```python
from build123d import *

# Parameters (mm, degrees)
SKETCH1_R           = 1.5
SKETCH1_R_2         = 7.5
SKETCH1_W           = 3
SKETCH1_H           = 10
BOSS_EXTRUDE1_DEPTH = 3


with BuildPart() as part:
    # Sketch1 → Boss-Extrude1 (new body)
    with BuildSketch(Plane.XY):
        with BuildLine():
            Line((-41.926461559, 19.115471746), (-34.926461559, -16.884528254))
            ThreePointArc((-34.926461559, -16.884528254), (-33.544217508, -19.207626568), (-31, -20.121049617))
            Line((-31, -20.121049617), (31, -20.121049617))
            ThreePointArc((31, -20.121049617), (33.544217508, -19.207626568), (34.926461559, -16.884528254))
            Line((34.926461559, -16.884528254), (41.926461559, 19.115471746))
            ThreePointArc((41.926461559, 19.115471746), (41.086576951, 22.42316789), (38, 23.878950383))
            Line((38, 23.878950383), (37.313708499, 23.878950383))
            ThreePointArc((37.313708499, 23.878950383), (35.004307422, 23.144936706), (33.542472333, 21.212283716))
            ThreePointArc((33.542472333, 21.212283716), (30.618802154, 17.346977735), (26, 15.878950383))
            Line((26, 15.878950383), (-26, 15.878950383))
            ThreePointArc((-26, 15.878950383), (-30.618802154, 17.346977735), (-33.542472333, 21.212283716))
            ThreePointArc((-33.542472333, 21.212283716), (-35.004307422, 23.144936706), (-37.313708499, 23.878950383))
            Line((-37.313708499, 23.878950383), (-38, 23.878950383))
            ThreePointArc((-38, 23.878950383), (-41.086576951, 22.42316789), (-41.926461559, 19.115471746))
        make_face()
        with Locations((38, 19.878950383)):
            Circle(SKETCH1_R, mode=Mode.SUBTRACT)
        with Locations((-38, 19.878950383)):
            Circle(SKETCH1_R, mode=Mode.SUBTRACT)
        with Locations((31, -16.121049617)):
            Circle(SKETCH1_R, mode=Mode.SUBTRACT)
        with Locations((-31, -16.121049617)):
            Circle(SKETCH1_R, mode=Mode.SUBTRACT)
        with Locations((0, 5.878950383)):
            Circle(SKETCH1_R_2, mode=Mode.SUBTRACT)
        with Locations((-27.5, 7.878950383)):
            Rectangle(SKETCH1_W, SKETCH1_H, mode=Mode.SUBTRACT)
        with Locations((-27.5, -12.121049617)):
            Rectangle(SKETCH1_W, SKETCH1_H, mode=Mode.SUBTRACT)
        with Locations((27.5, -12.121049617)):
            Rectangle(SKETCH1_W, SKETCH1_H, mode=Mode.SUBTRACT)
        with Locations((27.5, 7.878950383)):
            Rectangle(SKETCH1_W, SKETCH1_H, mode=Mode.SUBTRACT)
    extrude(amount=BOSS_EXTRUDE1_DEPTH)


solid = part.part
```
Here's how the part is built. I have some questions about the finished solid (model axes, mm). A direction names the side the tool comes from. Give positions to 0.01 mm unless a question says otherwise; leave off trailing zeros. Order: outer loops, then holes, each group sorted by start corner. A loop starts at its lowest first (then second) coordinate and runs counter-clockwise, first axis right, second up. Notation, with made-up numbers: (-29.5, 67) -> (1.5, 67) arc R26 cw to (1.5, 91) -> close; hole circle Ø4 at (23.25, -3.75). An arc over 180 degrees is marked (long way). Use CSV: the item, a comma, the result in double quotes. Start each with the question number.
Item 1: Suppose I cut it at C-C (x = 28). List the corners of the cut face in (y, z) for me, and give its area (3 significant figures).
Item 2: Suppose I cut it at B-B (y = -10). List the corners of the cut face in (x, z) for me, and give its area (3 significant figures).
Item 3: Suppose I cut it at D-D (y = 5). List the corners of the cut face in (x, z) for me, and give its area (3 significant figures).
Item 4: I'm going to push flat-ended pins straight in: P1, Ø1.5, axis at y = -13.5, z = 1.5, coming from the +X side; P2, Ø1.5, axis at y = -13.5, z = 2, coming from the -X side; P3, Ø0.9, axis at y = 9, z = 1, coming from the +X side. Where does each tip first touch, or does it pass through?
Item 5: On a 3-axis mill with a long thin cutter (end or side, diameter ignored), from which of +Z, -Z, +X, -X, +Y, -Y can I reach the whole of each face in a straight line? I mean faces 1 (the cylindrical face through (-33.574, -19.183, 1.479)), 2 (the cylindrical face through (-34.976, 23.125, 1.479)), 3 (the flat face through (-28, -17.121, 1)). Say none if no direction works.
Item 6: If I drill on probe 1 along X at (y, z) = (9.5, 2); probe 2 along X at (y, z) = (-8.5, 1); probe 3 along X at (y, z) = (-12, 0.8), over which ranges is the centre line in solid material (lowest first)? Write a range as [from, to].
Item 7: Thinking about a two-plate mould opening in X: for faces 4 (the cylindrical face through (33.514, -19.232, 1.479)), 5 (the flat face through (-1, -3, 3)), 6 (the cylindrical face through (-39.19, 18.966, 1.479)), 7 (the cylindrical face through (-41.055, 22.461, 1.479)), which applies, pulls with the +X half, pulls with the -X half, needs draft (parallel to the pull), parting line crosses it, or undercut?
Item 8: Suppose I cut it at A-A (x = 0). List the corners of the cut face in (y, z) for me, and give its area (3 significant figures).
Answer block:
1,outline,"(-20.12, 0) -> (-17.12, 0) -> (-17.12, 3) -> (-20.12, 3) -> close; (-7.12, 0) -> (2.88, 0) -> (2.88, 3) -> (-7.12, 3) -> close; (12.88, 0) -> (16.13, 0) -> (16.13, 3) -> (12.88, 3) -> close"
1,area,"48.8 mm^2"
2,outline,"(-36.27, 0) -> (-29, 0) -> (-29, 3) -> (-36.27, 3) -> close; (-26, 0) -> (26, 0) -> (26, 3) -> (-26, 3) -> close; (29, 0) -> (36.27, 0) -> (36.27, 3) -> (29, 3) -> close"
2,area,"200 mm^2"
3,outline,"(-39.18, 0) -> (-29, 0) -> (-29, 3) -> (-39.18, 3) -> close; (-26, 0) -> (-7.45, 0) -> (-7.45, 3) -> (-26, 3) -> close; (7.45, 0) -> (26, 0) -> (26, 3) -> (7.45, 3) -> close; (29, 0) -> (39.18, 0) -> (39.18, 3) -> (29, 3) -> close"
3,area,"172 mm^2"
4,P1,"stops at x = 35.73"
4,P2,"stops at x = -35.73"
4,P3,"stops at x = 40.05"
5,face 1,"+Z, -Z, -X, -Y"
5,face 2,"+Z, -Z, +Y"
5,face 3,"+Z, -Z"
6,probe 1,"x = [-40.06, -29], [-26, -6.57], [6.57, 26], [29, 40.06]"
6,probe 2,"x = [-36.56, -29], [-26, 26], [29, 36.56]"
6,probe 3,"x = [-35.88, -29], [-26, 26], [29, 35.88]"
7,face 4,"pulls with the +X half"
7,face 5,"needs draft"
7,face 6,"undercut"
7,face 7,"pulls with the -X half"
8,outline,"(-20.12, 0) -> (-1.62, 0) -> (-1.62, 3) -> (-20.12, 3) -> close; (13.38, 0) -> (15.88, 0) -> (15.88, 3) -> (13.38, 3) -> close"
8,area,"63.0 mm^2"
